from build123d import *

# Parameters (mm, degrees)
F1_DEPTH = 2.5
F2_R     = 6.9
F2_R_2   = 4.95
F2_R_3   = 3.325
F2_R_4   = 1.15
F3_DEPTH = 5.2
F4_R     = 7.275
F4_R_2   = 4.95
F5_DEPTH = 2.5
F6_SIZE2 = 2.49999
F6_SIZE  = 0.99999
F7_SIZE2 = 1
F7_SIZE  = 0.5


# Not quite as in the source:
# - a fillet or chamfer is up to 0.001 mm smaller than in the source, because OpenCascade refuses the exact size


with BuildPart() as f1:
    # F0 (on Top) → F1 (new body)
    with BuildSketch(Plane.XY):
        with BuildLine():
            Line((4.6819136376, 10.8858708742), (3.7330328633, 11.2466424164))
            ThreePointArc((3.7330328633, 11.2466424164), (-11.85, 0), (3.7330328633, -11.2466424164))
            Line((3.7330328633, -11.2466424164), (4.6819136376, -10.8858708742))
            ThreePointArc((4.6819136376, -10.8858708742), (9.8970494746, -6.5169710523), (11.85, 0))
            ThreePointArc((11.85, 0), (9.8970494746, 6.5169710523), (4.6819136376, 10.8858708742))
        make_face()
        with BuildLine():
            ThreePointArc((4.6819136376, 10.8858708742), (4.2113382884, 11.0764222482), (3.7330328633, 11.2466424164))
            Line((3.7330328633, 11.2466424164), (4.6819136376, 10.8858708742))
        make_face()
        with BuildLine():
            Line((4.6819136376, -10.8858708742), (3.7330328633, -11.2466424164))
            ThreePointArc((3.7330328633, -11.2466424164), (4.2113382884, -11.0764222482), (4.6819136376, -10.8858708742))
        make_face()
        with BuildLine():
            Line((20.2835521459, 4.9540116384), (4.6819136376, 10.8858708742))
            ThreePointArc((4.6819136376, 10.8858708742), (9.8970494746, 6.5169710523), (11.85, 0))
            ThreePointArc((11.85, 0), (9.8970494746, -6.5169710523), (4.6819136376, -10.8858708742))
            Line((4.6819136376, -10.8858708742), (20.2835521459, -4.9540116384))
            ThreePointArc((20.2835521459, -4.9540116384), (13.1, 0), (20.2835521459, 4.9540116384))
        make_face()
        with BuildLine():
            ThreePointArc((23.7, 0), (22.7630738232, 3.0089178808), (20.2835521459, 4.9540116384))
            ThreePointArc((20.2835521459, 4.9540116384), (13.1, 0), (20.2835521459, -4.9540116384))
            ThreePointArc((20.2835521459, -4.9540116384), (22.7630738232, -3.0089178808), (23.7, 0))
        make_face()
    extrude(amount=F1_DEPTH)

    # F2 (on Top) → F3 (join)
    with BuildSketch(Plane.XY):
        Circle(F2_R)
        Circle(F2_R_2, mode=Mode.SUBTRACT)
        with Locations((18.464056775, 0)):
            Circle(F2_R_3)
        with Locations((18.464056775, 0)):
            Circle(F2_R_4, mode=Mode.SUBTRACT)
    extrude(amount=-F3_DEPTH)

    # F4 (on face) → F5 (join)
    with BuildSketch(Plane(origin=(0, 0, -5.2), x_dir=(1, 0, 0), z_dir=(0, 0, -1))):
        Circle(F4_R)
        Circle(F4_R_2, mode=Mode.SUBTRACT)
    extrude(amount=F5_DEPTH)

    # F6 (size 1 and 2.5 in the source; OpenCascade refuses exactly that, so slightly less here)
    f6_edges = [f1.edges().sort_by_distance(p)[0] for p in [
        (-7.275, 0, -7.7),
    ]]
    f6_side = f1.faces().sort_by_distance((-7.069232, 0, -7.7))[0]
    chamfer(f6_edges, length=F6_SIZE, length2=F6_SIZE2, reference=f6_side)

    # F7
    f7_edges = [f1.edges().sort_by_distance(p)[0] for p in [
        (15.139057, 0, -5.2),
    ]]
    f7_side = f1.faces().sort_by_distance((15.233102, 0, -5.2))[0]
    chamfer(f7_edges, length=F7_SIZE, length2=F7_SIZE2, reference=f7_side)


solid = f1.part
Geometry check sheet. Reference: the model listing, model coordinates, mm. A direction names the side the tool comes from. Give positions to 0.01 mm unless a question says otherwise; leave off trailing zeros. Loops run counter-clockwise (first coordinate to the right, second up) from the corner with the lowest first, then second, coordinate; pieces in that order, holes last. Notation, with made-up numbers: (-28, -32.75) -> (2, -32.75) arc R18 cw to (2, -12.75) -> close; hole circle Ø2 at (21, -6.75). An arc over 180 degrees is marked (long way). Answer in a Markdown table with one row per item. Add a question column.
1) Gauge pin test, flat ends, axial feed: P1, Ø5, axis at y = 6.5, z = 1.5, coming from the -X side; P2, Ø6, axis at x = 19.5, y = -1, coming from the -Z side; P3, Ø9, axis at x = 0, y = 0, coming from the -Z side. Record the tip position at first contact, or that the pin passes through.
2) Set-up check for faces 1 (the face through (18, 0, 0)), 2 (the face through (5, -2, -7.7)), 3 (the face through (-0.9, 6.84, -2.56)), 4 (the face through (20, 0, -5.2)), 5 (the face through (6, 0, 2.5)): record each of +Z, -Z, +X, -X, +Y, -Y from which the full face is reachable in a straight line by a thin tool's end or side.
3) Material ranges on probe 1 along X at (y, z) = (0, -6.15) (3 decimals); probe 2 along X at (y, z) = (-2.5, -2); probe 3 along Z at (x, y) = (-3.5, -10.5), recorded low to high. Write a range as from..to.
4) Cross-section at D-D on x = 8. Record the boundary of the cut face in (y, z).
5) Cross-section at C-C on x = 12. Record the boundary of the cut face in (y, z), and give its area (3 significant figures).
6) Cross-section at B-B on z = 1. Record the boundary of the cut face in (x, y), and give its area (3 significant figures).
7) Draft check along Y on faces 6 (the face through (12.374, -7.961, 1.232)), 7 (the face through (21.636, 0.999, -2.071)), 8 (the face through (17.62, 0.78, -2.56)). Enter one of: pulls with the +Y half, pulls with the -Y half, needs draft (parallel to the pull), parting line crosses it, or undercut.
Outcome:
| question | item | result |
|---|---|---|
| 1 | P1 | stops at x = -11.15 |
| 1 | P2 | stops at z = -5.2 |
| 1 | P3 | stops at z = 0 |
| 2 | face 1 | -Z |
| 2 | face 2 | -Z, +X, -X, +Y, -Y |
| 2 | face 3 | none |
| 2 | face 4 | -Z, +X, +Y, -Y |
| 2 | face 5 | +Z, +X, -X, +Y, -Y |
| 3 | probe 1 | x = -6.895..-4.95, 4.95..6.895 |
| 3 | probe 2 | x = -6.43..-4.27, 4.27..6.43, 16.27..20.66 |
| 3 | probe 3 | z = 0..2.5 |
| 4 | outline | (-9.62, 0) -> (9.62, 0) -> (9.62, 2.5) -> (-9.62, 2.5) -> close |
| 5 | outline | (-8.1, 0) -> (8.1, 0) -> (8.1, 2.5) -> (-8.1, 2.5) -> close |
| 5 | area | 40.5 mm^2 |
| 6 | outline | (4.68, -10.89) -> (20.28, -4.95) arc R5.3 ccw to (20.28, 4.95) -> (4.68, 10.89) arc R11.85 ccw (long way) to start |
| 6 | area | 600 mm^2 |
| 7 | face 6 | pulls with the -Y half |
| 7 | face 7 | parting line crosses it |
| 7 | face 8 | undercut |
